from build123d import *

# Parameters (mm, degrees)
SKETCH1_W           = 71
SKETCH1_H           = 12.7
SKETCH1_R           = 2.75
BOSS_EXTRUDE1_DEPTH = 25.97
SKETCH2_W           = 19.05
SKETCH2_H           = 25.97
CUT_EXTRUDE1_DEPTH  = 4


with BuildPart() as part:
    # Sketch1 → Boss-Extrude1 (new body)
    with BuildSketch(Plane(origin=(0, 0, 0), x_dir=(1, 0, 0), z_dir=(0, 1, 0))):
        with Locations((25.5, 0)):
            Rectangle(SKETCH1_W, SKETCH1_H)
        with Locations(Location((0, 0, 0), (0, 0, 270))):
            Circle(SKETCH1_R, mode=Mode.SUBTRACT)
        with Locations(Location((51, 0, 0), (0, 0, 90))):
            Circle(SKETCH1_R, mode=Mode.SUBTRACT)
    extrude(amount=BOSS_EXTRUDE1_DEPTH)

    # Sketch2 → Cut-Extrude1 (cut)
    with BuildSketch(Plane(origin=(0, 0, -6.35), x_dir=(-1, 0, 0), z_dir=(0, 0, -1))):
        with Locations((-15.975, 12.985)):
            Rectangle(SKETCH2_W, SKETCH2_H)
    extrude(amount=-CUT_EXTRUDE1_DEPTH, mode=Mode.SUBTRACT)


solid = part.part
Design review of the part built by this model. Coordinates are the model's own, in mm. A direction names the side the tool comes from. Give positions to 0.01 mm unless a question says otherwise; leave off trailing zeros. Write each loop counter-clockwise with the first axis right and the second up, starting at its lowest first coordinate (ties: lowest second). Pieces come first, ordered by that corner, then holes. Notation, with made-up numbers: M -36.75,59 L -20.75,59 A33 cw -20.75,96 Z; hole C -20,41.25 d2. An arc over 180 degrees is marked long. Answer as a JSON object with one key per item and string values. Group by question number.
1) Tool access review of faces 1 (the face through (16, 13, -2.35)), 2 (the face through (-2, 13, -6.35)): name each direction out of +Z, -Z, +X, -X, +Y, -Y from which nothing blocks a thin tool from reaching the whole face with its end or side.
2) We need section B-B (z = -3.5). Give the boundary of the cut face in (x, y), and give its area (3 significant figures).
3) Clearance check with a flat-ended pin moving along its axis: pin 1 Ø9.5 at (x, y) = (19.5, 19) entering from -Z. State where the tip first meets the part, or that it passes through.
4) Mouldability with a two-part tool opening along X and no side actions: class faces 3 (the face through (43, 13, -6.35)), 4 (the face through (25.5, 13, -4)), 5 (the face through (-2.685, 12.803, -0.596)), 6 (the face through (-10, 13, 0)) as released by +X, released by -X, zero draft, split by the parting line, or undercut.
5) We need section D-D (z = 0). Give the boundary of the cut face in (x, y).
6) For line 1 along X through (y, z) = (20.5, 0); line 2 along X through (y, z) = (13, -4); line 3 along Z through (x, y) = (51, 19.25), list the stretches that pass through material, from the lowest coordinate up.
7) We need section A-A (x = 51). Give the boundary of the cut face in (y, z).
8) We need section C-C (y = 4.5). Give the boundary of the cut face in (x, z).
Answer key:
{
 "1": {"face 1": "-Z, +Y, -Y", "face 2": "-Z, +X, -X, +Y, -Y"},
 "2": {"outline": "M -10,0 L 6.45,0 L 6.45,25.97 L -10,25.97 Z; M 25.5,0 L 61,0 L 61,25.97 L 25.5,25.97 Z", "area": "1,350 mm²"},
 "3": {"pin 1": "stops at z = -2.35"},
 "4": {"face 3": "zero draft", "face 4": "undercut", "face 5": "undercut", "face 6": "released by -X"},
 "5": {"outline": "M -10,0 L -2.75,0 L -2.75,25.97 L -10,25.97 Z; M 2.75,0 L 48.25,0 L 48.25,25.97 L 2.75,25.97 Z; M 53.75,0 L 61,0 L 61,25.97 L 53.75,25.97 Z"},
 "6": {"line 1": "x = -10 to -2.75, 2.75 to 48.25, 53.75 to 61", "line 2": "x = -10 to 6.45, 25.5 to 61", "line 3": "z = -6.35 to -2.75, 2.75 to 6.35"},
 "7": {"outline": "M 0,-6.35 L 25.97,-6.35 L 25.97,-2.75 L 0,-2.75 Z; M 0,2.75 L 25.97,2.75 L 25.97,6.35 L 0,6.35 Z"},
 "8": {"outline": "M -10,-6.35 L 6.45,-6.35 L 6.45,-2.35 L 25.5,-2.35 L 25.5,-6.35 L 61,-6.35 L 61,6.35 L -10,6.35 Z; hole C 0,0 d5.5; hole C 51,0 d5.5"}
}
